Read the model definition and answer for the solid it produces. Units are mm, in the model's axes. Face numbers are marked on the shaded views. A direction names the side the tool comes from. Give positions to 0.01 mm unless a question says otherwise; leave off trailing zeros. Write each loop counter-clockwise with the first axis right and the second up, starting at its lowest first coordinate (ties: lowest second). Pieces come first, ordered by that corner, then holes. Notation, with made-up numbers: M 56.5,18 L 107.5,18 A30 ccw 107.5,49 Z; hole C 21.25,75 d3. An arc over 180 degrees is marked long. Use a Markdown table: item, result. Add a question column.
Item 1: A cutting plane is placed at B-B on z = 157. Determine the outline of the cut face in (x, y).
Item 2: Consider probe 1 along X at (y, z) = (334, 68); probe 2 along Y at (x, z) = (530.75, 157); probe 3 along Z at (x, y) = (407.5, 346). Determine where each line is inside the solid, lowest interval first. Write a range as [from, to].
Item 3: A cutting plane is placed at D-D on x = 432.5. Determine the outline of the cut face in (y, z).
Item 4: For the marked faces 1 and 2, determine the directions among +Z, -Z, +X, -X, +Y, -Y from which every point of the face is accessible in a straight line to the end or side of a thin tool.
Item 5: Given P1, Ø0.5, axis at x = 65.5, y = 357.5, coming from the +Z side; P2, Ø3, axis at x = 529, z = 92.5, coming from the -Y side; P3, Ø5, axis at y = 331, z = 141.5, coming from the +X side, each flat-ended and moving along its own axis, determine where each tip first touches the part or whether it passes through.
Item 6: A cutting plane is placed at A-A on x = 300. Determine the outline of the cut face in (y, z).
Item 7: The mould has two halves that part along X. Classify the marked faces 3, 4 and 5: pulls with the +X half, pulls with the -X half, needs draft (parallel to the pull), parting line crosses it, or undercut.
Item 8: A cutting plane is placed at C-C on z = 55.5. Determine the outline of the cut face in (x, y).
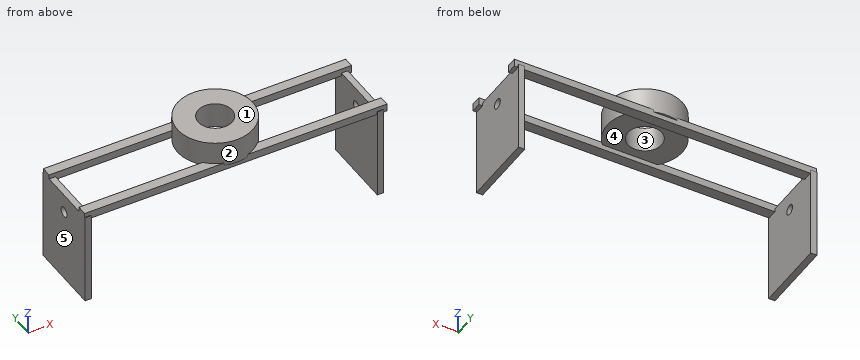
from build123d import *

# Parameters (mm, degrees)
SKETCH1_R           = 60
BOSS_EXTRUDE1_DEPTH = 40
SKETCH2_W           = 482
SKETCH2_H           = 16
BOSS_EXTRUDE2_DEPTH = 12
SKETCH3_W           = 482
SKETCH3_H           = 16
BOSS_EXTRUDE3_DEPTH = 12
SKETCH4_W           = 147
SKETCH4_H           = 116
BOSS_EXTRUDE4_DEPTH = 10
SKETCH5_W           = 147
SKETCH5_H           = 116
BOSS_EXTRUDE5_DEPTH = 10
SKETCH6_R           = 27
CUT_EXTRUDE1_DEPTH  = 210
SKETCH7_R           = 8
CUT_EXTRUDE2_DEPTH  = 502


with BuildPart() as part:
    # Sketch1 → Boss-Extrude1 (new body)
    with BuildSketch(Plane.XY.offset(190)):
        with Locations((300, 300)):
            Circle(SKETCH1_R)
    extrude(amount=BOSS_EXTRUDE1_DEPTH)

    # Sketch2 → Boss-Extrude2 (add)
    with BuildSketch(Plane.XY.offset(182)):
        with Locations((300, 349)):
            Rectangle(SKETCH2_W, SKETCH2_H)
    extrude(amount=BOSS_EXTRUDE2_DEPTH)

    # Sketch3 → Boss-Extrude3 (add)
    with BuildSketch(Plane.XY.offset(182)):
        with Locations((300, 251)):
            Rectangle(SKETCH3_W, SKETCH3_H)
    extrude(amount=BOSS_EXTRUDE3_DEPTH)

    # Sketch4 → Boss-Extrude4 (add)
    with BuildSketch(Plane(origin=(525, 0, 0), x_dir=(0, 0, -1), z_dir=(1, 0, 0))):
        with Locations((-113.5, 300)):
            Rectangle(SKETCH4_W, SKETCH4_H)
    extrude(amount=BOSS_EXTRUDE4_DEPTH)

    # Sketch5 → Boss-Extrude5 (add)
    with BuildSketch(Plane(origin=(59, 0, 0), x_dir=(0, 0, -1), z_dir=(1, 0, 0))):
        with Locations((-113.5, 300)):
            Rectangle(SKETCH5_W, SKETCH5_H)
    extrude(amount=BOSS_EXTRUDE5_DEPTH)

    # Sketch6 → Cut-Extrude1 (cut)
    with BuildSketch(Plane.XY.offset(230)):
        with Locations((300, 300)):
            Circle(SKETCH6_R)
    extrude(amount=-CUT_EXTRUDE1_DEPTH, mode=Mode.SUBTRACT)

    # Sketch7 → Cut-Extrude2 (cut)
    with BuildSketch(Plane(origin=(535, 0, 0), x_dir=(0, 0, -1), z_dir=(1, 0, 0))):
        with Locations((-157, 300)):
            Circle(SKETCH7_R)
    extrude(amount=-CUT_EXTRUDE2_DEPTH, mode=Mode.SUBTRACT)


solid = part.part
Filled in:
| question | item | result |
|---|---|---|
| 1 | outline | M 59,242 L 69,242 L 69,292 L 59,292 Z; M 59,308 L 69,308 L 69,358 L 59,358 Z; M 525,242 L 535,242 L 535,292 L 525,292 Z; M 525,308 L 535,308 L 535,358 L 525,358 Z |
| 2 | probe 1 | [59, 69], [525, 535] |
| 2 | probe 2 | [242, 292], [308, 358] |
| 2 | probe 3 | [182, 194] |
| 3 | outline | M 243,182 L 259,182 L 259,194 L 243,194 Z; M 341,182 L 357,182 L 357,194 L 341,194 Z |
| 4 | face 1 | +Z, +X, -X, +Y, -Y |
| 4 | face 2 | +Z |
| 5 | P1 | z = 187 |
| 5 | P2 | y = 242 |
| 5 | P3 | x = 535 |
| 6 | outline | M 240,190 L 243,190 L 243,182 L 259,182 L 259,190 L 273,190 L 273,230 L 240,230 Z; M 327,190 L 341,190 L 341,182 L 357,182 L 357,190 L 360,190 L 360,230 L 327,230 Z |
| 7 | face 3 | undercut |
| 7 | face 4 | needs draft |
| 7 | face 5 | pulls with the -X half |
| 8 | outline | M 59,242 L 69,242 L 69,358 L 59,358 Z; M 525,242 L 535,242 L 535,358 L 525,358 Z |
